from build123d import *

# Parameters (mm, degrees)
SKETCH1_W           = 66
SKETCH1_H           = 53
BOSS_EXTRUDE1_DEPTH = 26
SHELL1_T            = -1.6
FILLET1_R           = 2
SKETCH2_R           = 2.5
SKETCH2_W           = 16
SKETCH2_H           = 28
CUT_EXTRUDE1_DEPTH  = 5
SKETCH3_R           = 2
BOSS_EXTRUDE2_DEPTH = 24.4
FILLET2_R           = 3
FILLET3_R           = 1.5
SKETCH4_R           = 1
CUT_EXTRUDE2_DEPTH  = 515.754449712


with BuildPart() as part:
    # Sketch1 → Boss-Extrude1 (new body)
    with BuildSketch(Plane.XY.offset(40)):
        with Locations((106.004254286, 468.448442556)):
            Rectangle(SKETCH1_W, SKETCH1_H)
    extrude(amount=BOSS_EXTRUDE1_DEPTH)

    # Shell1
    shell1_openings = [part.faces().sort_by_distance(p)[0] for p in [
        (106.004254286, 468.448442556, 66),
    ]]
    offset(amount=SHELL1_T, openings=shell1_openings, kind=Kind.INTERSECTION)

    # Fillet1
    fillet1_edges = [part.edges().sort_by_distance(p)[0] for p in [
        (73.004254286, 494.948442556, 53),
        (139.004254286, 494.948442556, 53),
        (139.004254286, 441.948442556, 53),
        (73.004254286, 441.948442556, 53),
    ]]
    fillet(fillet1_edges, radius=FILLET1_R)

    # Sketch2 → Cut-Extrude1 (cut)
    with BuildSketch(Plane.XY.offset(41.6)):
        with Locations((79.932206481, 485.091899203)):
            Circle(SKETCH2_R)
        with Locations((132.121487701, 485.091899203)):
            Circle(SKETCH2_R)
        with Locations((121.980911954, 461.997551837)):
            Rectangle(SKETCH2_W, SKETCH2_H)
        with Locations((89.980911954, 461.997551837)):
            Rectangle(SKETCH2_W, SKETCH2_H)
    extrude(amount=-CUT_EXTRUDE1_DEPTH, mode=Mode.SUBTRACT)

    # Sketch3 → Boss-Extrude2 (add)
    with BuildSketch(Plane.XY.offset(41.6)):
        with Locations((89.997613128, 492.01389561)):
            Circle(SKETCH3_R)
        with Locations((121.954957607, 492.01389561)):
            Circle(SKETCH3_R)
        with Locations((75.98529147, 445.090629457)):
            Circle(SKETCH3_R)
        with Locations((135.997102491, 445.090629457)):
            Circle(SKETCH3_R)
    extrude(amount=BOSS_EXTRUDE2_DEPTH)

    # Fillet2
    fillet2_edges = [part.edges().sort_by_distance(p)[0] for p in [
        (88.507987521, 493.348442556, 53.8),
        (91.487238734, 493.348442556, 53.8),
        (120.465332, 493.348442556, 53.8),
        (123.444583213, 493.348442556, 53.8),
        (134.723658514, 443.548442556, 53.8),
        (137.404254286, 446.5118697, 53.8),
        (77.258735447, 443.548442556, 53.8),
        (74.604254286, 446.537258746, 53.8),
    ]]
    fillet(fillet2_edges, radius=FILLET2_R)

    # Fillet3
    fillet3_edges = [part.edges().sort_by_distance(p)[0] for p in [
        (81.980911954, 447.997551837, 40.8),
        (81.980911954, 475.997551837, 40.8),
        (97.980911954, 475.997551837, 40.8),
        (97.980911954, 447.997551837, 40.8),
        (113.980911954, 475.997551837, 40.8),
        (129.980911954, 475.997551837, 40.8),
        (129.980911954, 447.997551837, 40.8),
        (113.980911954, 447.997551837, 40.8),
    ]]
    fillet(fillet3_edges, radius=FILLET3_R)

    # Sketch4 → Cut-Extrude2 (cut, through all)
    with BuildSketch(Plane.XY.offset(66)):
        with Locations((89.975104107, 492.043680815)):
            Circle(SKETCH4_R)
        with Locations((122.005633098, 492.043680815)):
            Circle(SKETCH4_R)
        with Locations((75.994176926, 444.994296882)):
            Circle(SKETCH4_R)
        with Locations((136.02065658, 444.994296882)):
            Circle(SKETCH4_R)
    extrude(amount=-CUT_EXTRUDE2_DEPTH, mode=Mode.SUBTRACT)


solid = part.part
CAD build for the part. Positions are in the model's coordinates, mm. A direction names the side the tool comes from. Give positions to 0.01 mm unless a question says otherwise; leave off trailing zeros. Order: outer loops, then holes, each group sorted by start corner. A loop starts at its lowest first (then second) coordinate and runs counter-clockwise, first axis right, second up. Notation, with made-up numbers: (45.25, 71.25) - (72.25, 71.25) arc R18 cw to (72.25, 99.25) - close; hole circle Ø9 at (8, 34.25). An arc over 180 degrees is marked (long way). Answer in a Markdown table with one row per item.
1. Saw through at C-C, the plane x = 125.5. Give the cut face in (y, z), plus the area to 3 significant figures.
Data:
| item | result |
|---|---|
| outline | (441.95, 40) - (448, 40) - (448, 41.6) - (443.55, 41.6) - (443.55, 66) - (441.95, 66) - close; (476, 40) - (494.95, 40) - (494.95, 66) - (493.11, 66) - (493.11, 41.6) - (476, 41.6) - close |
| area | 124 mm² |
2. Saw through at A-A, the plane y = 458.5. Give the cut face in (x, z).
Data:
| item | result |
|---|---|
| outline | (73, 40) - (81.98, 40) - (81.98, 41.6) - (74.6, 41.6) - (74.6, 66) - (73, 66) - close; (97.98, 40) - (113.98, 40) - (113.98, 41.6) - (97.98, 41.6) - close; (129.98, 40) - (139, 40) - (139, 66) - (137.4, 66) - (137.4, 41.6) - (129.98, 41.6) - close |
3. Tool access for faces 5 (the cylindrical face through (129.53, 448.425, 40.789)), 6 (the flat face through (132, 493.348, 54)), 7 (the flat face through (106, 443, 66)): list every direction of +Z, -Z, +X, -X, +Y, -Y with a clear straight run to the whole face (end or side of a thin tool).
Data:
| item | result |
|---|---|
| face 5 | +Z, -Z |
| face 6 | +Z |
| face 7 | +Z, +X, -X, +Y, -Y |
4. Saw through at B-B, the plane x = 102.5. Give the cut face in (y, z), plus the area to 3 significant figures.
Data:
| item | result |
|---|---|
| outline | (441.95, 40) - (494.95, 40) - (494.95, 66) - (493.35, 66) - (493.35, 41.6) - (443.55, 41.6) - (443.55, 66) - (441.95, 66) - close |
| area | 163 mm² |
5. Saw through at D-D, the plane y = 479.5. Give the cut face in (x, z).
Data:
| item | result |
|---|---|
| outline | (73, 40) - (139, 40) - (139, 66) - (137.4, 66) - (137.4, 41.6) - (74.6, 41.6) - (74.6, 66) - (73, 66) - close |
6. Pull direction X, two halves, no side cores. Call faces 1 (the cylindrical face through (73.575, 442.55, 53.182)), 2 (the flat face through (106, 441.948, 53)), 3 (the flat face through (106, 443.548, 54)), 4 (the flat face through (81.981, 462, 41)): pulls with the +X half, pulls with the -X half, needs draft (parallel to the pull), parting line crosses it, or undercut.
Data:
| item | result |
|---|---|
| face 1 | pulls with the -X half |
| face 2 | needs draft |
| face 3 | undercut |
| face 4 | undercut |
7. Probe probe 1 along Y at (x, z) = (97, 42.5); probe 2 along Y at (x, z) = (131.5, 56); probe 3 along X at (y, z) = (483.5, 56.5). List the from-to ranges inside material, lowest first. Write a range as [from, to].
Data:
| item | result |
|---|---|
| probe 1 | y = [441.95, 443.55], [493.35, 494.95] |
| probe 2 | y = [441.95, 443.56], [493.35, 494.95] |
| probe 3 | x = [73, 74.6], [137.4, 139] |
8. Flat gauge pins, fed straight in: pin 1 (2 mm diameter, centred on x = 99.5, y = 483.5, fed in from +Z); pin 2 (1.2 mm diameter, centred on x = 89.98, y = 492.04, fed in from -Z). Where does each tip first touch, or does it go through?
Data:
| item | result |
|---|---|
| pin 1 | stops at z = 41.6 |
| pin 2 | passes through |
